Source: three-view drawing plus pictorial views. Frame: mm from the lowest corner of the part. Coordinates: 2 decimals unless noted, no trailing zeros. Order: outer loops, then holes, each group sorted by start corner. A loop starts at its lowest first (then second) coordinate and runs counter-clockwise, first axis right, second up. Notation, with made-up numbers: (31.25, -13) - (64.25, -13) arc R20 cw to (64.25, 26) - close; hole circle Ø7 at (-35.5, 7.5). An arc over 180 degrees is marked (long way). One line per question, with ' | ' between items.
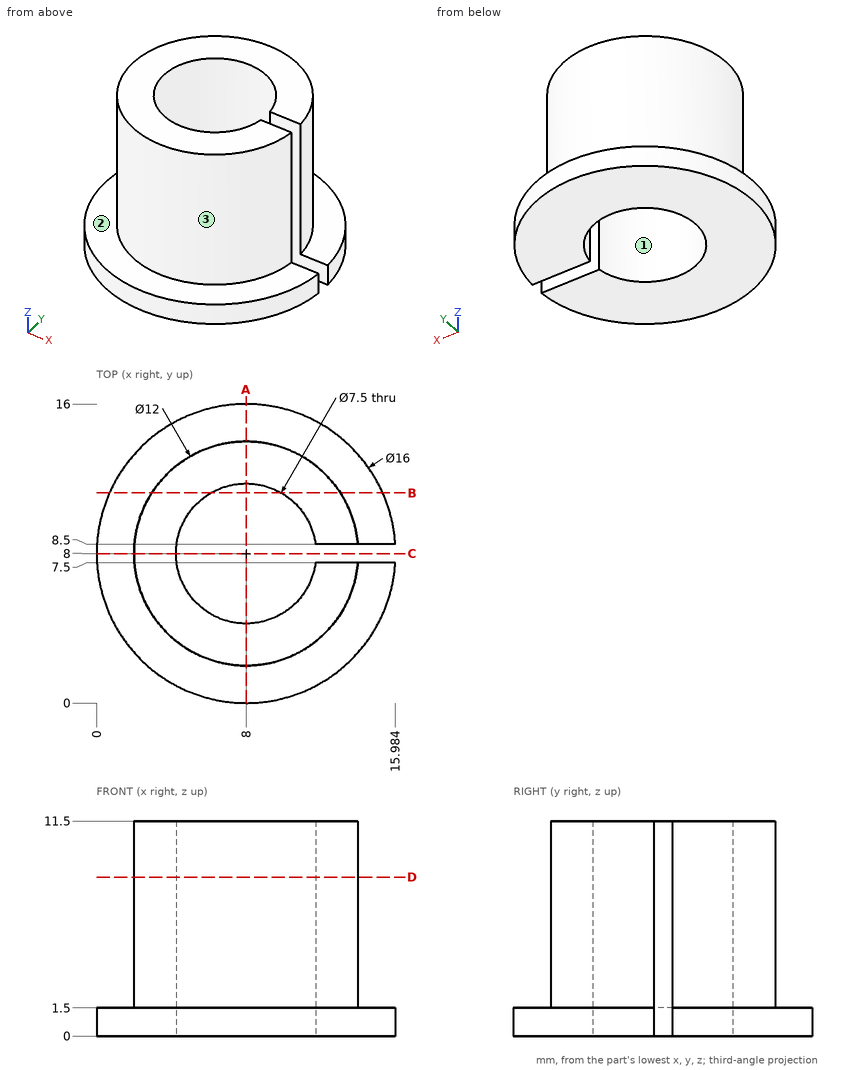
Item 1: Section D-D on z = 8.5. Return the cut outline in (x, y).
Data:
outline: (11.72, 7.5) arc R3.75 cw (long way) to (11.72, 8.5) - (13.98, 8.5) arc R6 ccw (long way) to (13.98, 7.5) - close
Item 2: Contact query for flat-ended pins moving along their axis: P1, Ø6, axis at x = 4.5, z = 8, coming from the -Y side; P2, Ø1, axis at y = 8.5, z = 10, coming from the +X side; P3, Ø2, axis at x = 13, z = 7.5, coming from the -Y side. Output: stop coordinate, or through.
Data:
P1: y = 2.02 | P2: x = 13.98 | P3: y = 3.53
Item 3: Section C-C on y = 8. Return the cut outline in (x, z), and give its area (3 significant figures).
Data:
outline: (0, 0) - (4.25, 0) - (4.25, 11.5) - (2, 11.5) - (2, 1.5) - (0, 1.5) - close | area: 28.9 mm^2
Item 4: Section A-A on x = 8. Return the cut outline in (y, z).
Data:
outline: (0, 0) - (4.25, 0) - (4.25, 11.5) - (2, 11.5) - (2, 1.5) - (0, 1.5) - close; (11.75, 0) - (16, 0) - (16, 1.5) - (14, 1.5) - (14, 11.5) - (11.75, 11.5) - close
Item 5: Section B-B on y = 11.25. Return the cut outline in (x, z).
Data:
outline: (0.69, 0) - (6.13, 0) - (6.13, 11.5) - (2.96, 11.5) - (2.96, 1.5) - (0.69, 1.5) - close; (9.87, 0) - (15.31, 0) - (15.31, 1.5) - (13.04, 1.5) - (13.04, 11.5) - (9.87, 11.5) - close
Item 6: Ray query, line 1 (Y direction, x = 8, z = 3.5); line 2 (Y direction, x = 8, z = 1); line 3 (X direction, y = 8, z = 8.5). Return the intervals inside material, ascending.
Data:
line 1: 2 to 4.25, 11.75 to 14 | line 2: 0 to 4.25, 11.75 to 16 | line 3: 2 to 4.25
Item 7: Draft query along X for the marked faces 1, 2 and 3. Return one class per face: released by +X, released by -X, zero draft, split by the parting line, or undercut.
Data:
face 1: undercut | face 2: zero draft | face 3: split by the parting line
